```python
from build123d import *

# Parameters (mm, degrees)
SKETCH_1_W          = 360
SKETCH_1_H          = 300
EXTRUDE_1_DEPTH     = 4
SKETCH_2_W          = 260
SKETCH_2_H          = 30
CUT_EXTRUDE_1_DEPTH = 469.632051827
SKETCH_3_W          = 30
SKETCH_3_H          = 115
CUT_EXTRUDE_2_DEPTH = 469.632051827
CUT_EXTRUDE_3_DEPTH = 469.632051827
CUT_EXTRUDE_4_DEPTH = 330.611201771
CUT_EXTRUDE_5_DEPTH = 330.611201771


with BuildPart() as part:
    # 草图1 → 凸台-拉伸1 (new body)
    with BuildSketch(Plane(origin=(0, 0, 0), x_dir=(1, 0, 0), z_dir=(0, 1, 0))):
        with Locations((180, -150)):
            Rectangle(SKETCH_1_W, SKETCH_1_H)
    extrude(amount=EXTRUDE_1_DEPTH)

    # 草图2 → 切除-拉伸1 (cut, through all)
    with BuildSketch(Plane(origin=(0, 4, 0), x_dir=(1, 0, 0), z_dir=(0, 1, 0))):
        with Locations((180, -15)):
            Rectangle(SKETCH_2_W, SKETCH_2_H)
        Polygon((310, -270), (50, -270), (50, -300), (310, -300), (310, -297.414750004), align=None)
    extrude(amount=-CUT_EXTRUDE_1_DEPTH, mode=Mode.SUBTRACT)

    # 草图3 → 切除-拉伸2 (cut, through all)
    with BuildSketch(Plane(origin=(0, 4, 0), x_dir=(1, 0, 0), z_dir=(0, 1, 0))):
        with Locations((15, -152.5)):
            Rectangle(SKETCH_3_W, SKETCH_3_H)
        with Locations((345, -152.5)):
            Rectangle(SKETCH_3_W, SKETCH_3_H)
    extrude(amount=-CUT_EXTRUDE_2_DEPTH, mode=Mode.SUBTRACT)

    # 草图4 → 切除-拉伸3 (cut, through all)
    with BuildSketch(Plane(origin=(0, 4, 0), x_dir=(1, 0, 0), z_dir=(0, 1, 0))):
        with BuildLine():
            ThreePointArc((136.482762036, -30), (73.799150344, -77.524140336), (50, -152.5))
            Line((50, -152.5), (180, -152.5))
            Line((180, -152.5), (180, -30))
            Line((180, -30), (136.482762036, -30))
        make_face()
        with BuildLine():
            Line((180, -30), (180, -152.5))
            Line((180, -152.5), (310, -152.5))
            ThreePointArc((310, -152.5), (286.200849656, -77.524140336), (223.517237964, -30))
            Line((223.517237964, -30), (180, -30))
        make_face()
        with BuildLine():
            Line((180, -152.5), (50, -152.5))
            ThreePointArc((50, -152.5), (70.157400056, -222.031311203), (124.378511347, -270))
            Line((124.378511347, -270), (180, -270))
            Line((180, -270), (180, -152.5))
        make_face()
        with BuildLine():
            Line((310, -152.5), (180, -152.5))
            Line((180, -152.5), (180, -270))
            Line((180, -270), (235.621488653, -270))
            ThreePointArc((235.621488653, -270), (289.842599944, -222.031311203), (310, -152.5))
        make_face()
    extrude(amount=-CUT_EXTRUDE_3_DEPTH, mode=Mode.SUBTRACT)


with BuildPart() as cut_extrude_3_kept_piece:
    # of the separate pieces the step leaves, the one the design keeps (cut_extrude_3_pieces_kept)
    add(part.part.solids().sort_by_distance((0, 0, 0))[0])

    # 草图5 → 切除-拉伸4 (cut, through all)
    with BuildSketch(Plane(origin=(0, 4, 0), x_dir=(1, 0, 0), z_dir=(0, 1, 0))):
        with BuildLine():
            ThreePointArc((15, -27.25), (12.25, -30), (15, -32.75))
            Line((15, -32.75), (15, -30))
            Line((15, -30), (15, -27.25))
        make_face()
        with BuildLine():
            Line((15, -30), (15, -32.75))
            ThreePointArc((15, -32.75), (16.944543648, -31.944543648), (17.75, -30))
            ThreePointArc((17.75, -30), (16.944543648, -28.055456352), (15, -27.25))
            Line((15, -27.25), (15, -30))
        make_face()
        with BuildLine():
            ThreePointArc((15, -60.994001195), (12.25, -63.744001195), (15, -66.494001195))
            Line((15, -66.494001195), (15, -63.744001195))
            Line((15, -63.744001195), (15, -60.994001195))
        make_face()
        with BuildLine():
            Line((15, -63.744001195), (15, -66.494001195))
            ThreePointArc((15, -66.494001195), (16.944543648, -65.688544844), (17.75, -63.744001195))
            ThreePointArc((17.75, -63.744001195), (16.944543648, -61.799457547), (15, -60.994001195))
            Line((15, -60.994001195), (15, -63.744001195))
        make_face()
        with BuildLine():
            ThreePointArc((15, -237.25), (12.25, -240), (15, -242.75))
            Line((15, -242.75), (15, -240))
            Line((15, -240), (15, -237.25))
        make_face()
        with BuildLine():
            Line((15, -240), (15, -242.75))
            ThreePointArc((15, -242.75), (16.944543648, -241.944543648), (17.75, -240))
            ThreePointArc((17.75, -240), (16.944543648, -238.055456352), (15, -237.25))
            Line((15, -237.25), (15, -240))
        make_face()
        with BuildLine():
            ThreePointArc((15, -267.25), (12.25, -270), (15, -272.75))
            Line((15, -272.75), (15, -270))
            Line((15, -270), (15, -267.25))
        make_face()
        with BuildLine():
            Line((15, -270), (15, -272.75))
            ThreePointArc((15, -272.75), (16.944543648, -271.944543648), (17.75, -270))
            ThreePointArc((17.75, -270), (16.944543648, -268.055456352), (15, -267.25))
            Line((15, -267.25), (15, -270))
        make_face()
    extrude(amount=-CUT_EXTRUDE_4_DEPTH, mode=Mode.SUBTRACT)

    # 草图6 → 切除-拉伸5 (cut, through all)
    with BuildSketch(Plane(origin=(0, 4, 0), x_dir=(1, 0, 0), z_dir=(0, 1, 0))):
        with BuildLine():
            Line((50, -50), (66.378679656, -50))
            ThreePointArc((66.378679656, -50), (67.764498955, -50.925974851), (67.439339828, -52.560660172))
            Line((67.439339828, -52.560660172), (42.560660172, -77.439339828))
            ThreePointArc((42.560660172, -77.439339828), (40.925974851, -77.764498955), (40, -76.378679656))
            Line((40, -76.378679656), (40, -51.5))
            ThreePointArc((40, -51.5), (40.439339828, -50.439339828), (41.5, -50))
            Line((41.5, -50), (50, -50))
        make_face()
    cut_extrude_5 = extrude(amount=-CUT_EXTRUDE_5_DEPTH, mode=Mode.SUBTRACT)

    # 镜向1: 切除-拉伸5 across plane
    add(cut_extrude_5.mirror(Plane.XY.offset(150)), mode=Mode.SUBTRACT)


solid = cut_extrude_3_kept_piece.part
```
Geometry check sheet. Reference: the model listing, model coordinates, mm. A direction names the side the tool comes from. Give positions to 0.01 mm unless a question says otherwise; leave off trailing zeros. Order: outer loops, then holes, each group sorted by start corner. A loop starts at its lowest first (then second) coordinate and runs counter-clockwise, first axis right, second up.
1. Access from +Z, -Z, +X, -X, +Y, -Y to the whole of each face (thin tool, end or side, straight path). Record for faces 3 (the face through (55, 2, 65)), 4 (the face through (37, 0, 148)).
2. Release check for a two-part mould opening along Z. For faces 1 (the face through (55, 2, 235)), 2 (the face through (37, 4, 148)) record: pulls with the +Z half, pulls with the -Z half, needs draft (parallel to the pull), parting line crosses it, or undercut.
3. Gauge pin test, flat ends, axial feed: pin 1 Ø2 at (x, y) = (72, 2.5) entering from +Z; pin 2 Ø2 at (y, z) = (2, 238) entering from +X; pin 3 Ø1.2 at (y, z) = (2, 11.5) entering from +X. Record the tip position at first contact, or that the pin passes through.
4. Section check B-B, the plane y = 3.2. Enter the section's corners in (x, z).
5. Section check C-C, the plane z = 167.5. Enter the section's corners in (x, y), and give its area (3 significant figures).
6. Section check D-D, the plane x = 128. Enter the section's corners in (y, z).
7. Thickness scan on L1, parallel to Z at x = 10.5, y = 3.65; L2, parallel to Z at x = 14, y = 3.8; L3, parallel to X at y = 0.7, z = 64. Record the ranges inside material, lowest first.
8. Section check A-A, the plane x = 106. Enter the section's corners in (y, z), and give its area (3 significant figures).
Values follow:
1. face 3: +Y, -Y
1. face 4: +Z, -Z, +X, -X, -Y
2. face 1: undercut
2. face 2: needs draft
3. pin 1: stops at z = 270
3. pin 2: stops at x = 82.95
3. pin 3: stops at x = 50
4. outline: (0, 0) - (50, 0) - (50, 30) - (136.48, 30) arc R130 cw to (124.38, 270) - (50, 270) - (50, 300) - (0, 300) - (0, 210) - (30, 210) - (30, 95) - (0, 95) - close; hole circle Ø5.5 at (15, 30); hole circle Ø5.5 at (15, 63.74); hole circle Ø5.5 at (15, 240); hole circle Ø5.5 at (15, 270); hole (40, 51.5) arc R1.5 ccw to (41.5, 50) - (66.38, 50) arc R1.5 ccw to (67.44, 52.56) - (42.56, 77.44) arc R1.5 ccw to (40, 76.38) - close; hole (40, 223.62) arc R1.5 ccw to (42.56, 222.56) - (67.44, 247.44) arc R1.5 ccw to (66.38, 250) - (41.5, 250) arc R1.5 ccw to (40, 248.5) - close
5. outline: (30, 0) - (50.87, 0) - (50.87, 4) - (30, 4) - close
5. area: 83.5 mm2
6. outline: (0, 30) - (4, 30) - (4, 33.35) - (0, 33.35) - close
7. L1: z = 0 to 95, 210 to 300
7. L2: z = 0 to 27.44, 32.56 to 61.18, 66.31 to 95, 210 to 237.44, 242.56 to 267.44, 272.56 to 300
7. L3: x = 0 to 12.26, 17.74 to 40, 56 to 84.78
8. outline: (0, 30) - (4, 30) - (4, 45.62) - (0, 45.62) - close; (0, 259.38) - (4, 259.38) - (4, 270) - (0, 270) - close
8. area: 105 mm2
